Build history of the part. All positions in model axes, mm. Face numbers are marked on the shaded views. A direction names the side the tool comes from. Coordinates: 2 decimals unless noted, no trailing zeros. Write each loop counter-clockwise with the first axis right and the second up, starting at its lowest first coordinate (ties: lowest second). Pieces come first, ordered by that corner, then holes.
Autodesk Inventor part; units mm, degrees
ref_plane "YZ Plane" through (0, 0, 0) normal (1, 0, 0) x (0, 1, 0)
ref_plane "XZ Plane" through (0, 0, 0) normal (0, 1, 0) x (-1, 0, 0)
ref_plane "XY Plane" through (0, 0, 0) normal (0, 0, 1) x (1, 0, 0)
sketch "Sketch1" plane through (0, 0, 0) normal (0, 0, 1) x (1, 0, 0)
  point P0 (0, 0)
sketch "Sketch2" plane through (0, 0, 0) normal (0, 0, 1) x (1, 0, 0)
  line L0 (-50, -25) -> (50, -25)
  line L1 (50, -25) -> (50, 25)
  line L2 (50, 25) -> (-50, 25)
  line L3 (-50, 25) -> (-50, -25)
  line L4 (-50, -25) -> (50, 25) construction
  line L5 (50, -25) -> (-50, 25) construction
  line L6 (-55, -30) -> (55, -30)
  line L7 (55, -30) -> (55, 30)
  line L8 (55, 30) -> (-55, 30)
  line L9 (-55, 30) -> (-55, -30)
  line L10 (-55, -30) -> (55, 30) construction
  line L11 (55, -30) -> (-55, 30) construction
  point P0 (0, 0)
  dimension "d0" = 100
  dimension "d1" = 50
  dimension "d2" = 110
  dimension "d3" = 60
sketch "Sketch3" plane through (0, 0, 0) normal (1, 0, 0) x (0, 1, 0)
  line L0 (0, 0) -> (0, -75)
  arc A0 (0, -75) -> (100, -175) centre (100, -75) ccw
  line L1 (100, -75) -> (100, -175) construction
  line L2 (100, -75) -> (0, -75) construction
  line L3 (100, -175) -> (150, -175)
sweep "Sweep1" add profiles "Sketch2" path "Sketch3"
sketch "Sketch4" plane through (-55, -30, 0) normal (0, -1, 0) x (1, 0, 0)
  circle A0 centre (55, -37.5) radius 3.5
  point P0 (55, 0)
  dimension "d9" = 7
extrude "Extrusion1" cut sketch "Sketch4" against normal blind 10
chamfer "Chamfer1" distance 5 angle 45 1 edges at (-3.5, -25, -37.5)
properties part number "RecTubeNewTappingChamfer"
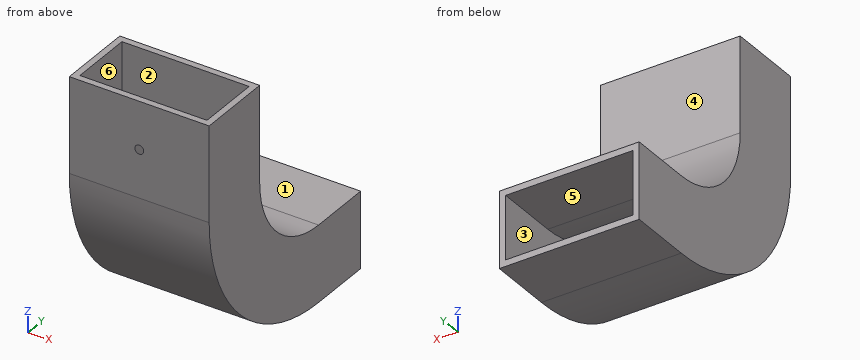
1. Saw through at C-C on y = 127.5. List the corners of the cut face in (x, z), plus the area to 3 significant figures.
Computed values:
outline: (-55, -205) - (55, -205) - (55, -145) - (-55, -145) - close; hole (-50, -200) - (50, -200) - (50, -150) - (-50, -150) - close
area: 1,600 mm2
2. Mould opens along Z. For the marked faces 1, 2 and 3 say: +Z half, -Z half, draft (parallel to the pull), parting line (faces both ways), or undercut.
Computed values:
face 1: +Z half
face 2: draft
face 3: undercut
3. Saw through at A-A on x = 11.5. List the corners of the cut face in (y, z), plus the area to 3 significant figures.
Computed values:
outline: (-30, -75) arc R130 ccw to (100, -205) - (150, -205) - (150, -200) - (100, -200) arc R125 cw to (-25, -75) - (-25, 0) - (-30, 0) - close; (25, -75) arc R75 ccw to (100, -150) - (150, -150) - (150, -145) - (100, -145) arc R70 cw to (30, -75) - (30, 0) - (25, 0) - close
area: 2,820 mm2
4. 3-axis set-ups, long thin cutter, end or side, ignore diameter. For the marked faces 4, 5 and 6: which of +Z, -Z, +X, -X, +Y, -Y reach the whole face in a straight line?
Computed values:
face 4: +Z, +X, -X, +Y
face 5: +Y
face 6: none
5. Saw through at B-B on z = -53. List the corners of the cut face in (x, y), plus the area to 3 significant figures.
Computed values:
outline: (-55, -30) - (55, -30) - (55, 30) - (-55, 30) - close; hole (-50, -25) - (50, -25) - (50, 25) - (-50, 25) - close
area: 1,600 mm2
6. Flat gauge pins, fed straight in: pin 1 (1.5 mm diameter, centred on x = -41, y = 15.5, fed in from +Z); pin 2 (12 mm diameter, centred on x = -41, y = 55.5, fed in from +Z); pin 3 (10 mm diameter, centred on x = -25.5, y = 110, fed in from +Z). Where does each tip first touch, or does it go through?
Computed values:
pin 1: stops at z = -166.42
pin 2: stops at z = -123.47
pin 3: stops at z = -145
7. Saw through at D-D on x = 0. State how many separate pieces and enclosed holes the cut face has, plus the area to 3 significant figures.
Computed values:
separate pieces: 3
enclosed holes: 0
area: 2,760 mm2
8. Probe line 1 along Z through (x, y) = (-6.5, 109.5); line 2 along X through (y, z) = (3.5, -21); line 3 along Y through (x, z) = (-34, -37). List the from-to ranges inside material, lowest first.
Computed values:
line 1: z = -205 to -200, -150 to -145
line 2: x = -55 to -50, 50 to 55
line 3: y = -30 to -25, 25 to 30
